For this review, use the dimensioned drawing (mm, ordinates from the lowest corner) and the shaded views. Give positions to 0.01 mm unless a question says otherwise; leave off trailing zeros. Write each loop counter-clockwise with the first axis right and the second up, starting at its lowest first coordinate (ties: lowest second). Pieces come first, ordered by that corner, then holes. Notation, with made-up numbers: (87.5, -7) -> (140.5, -7) arc R17 ccw to (140.5, 17) -> close; hole circle Ø5 at (81.5, 27.25). An arc over 180 degrees is marked (long way). Answer as CSV lines item,"result".
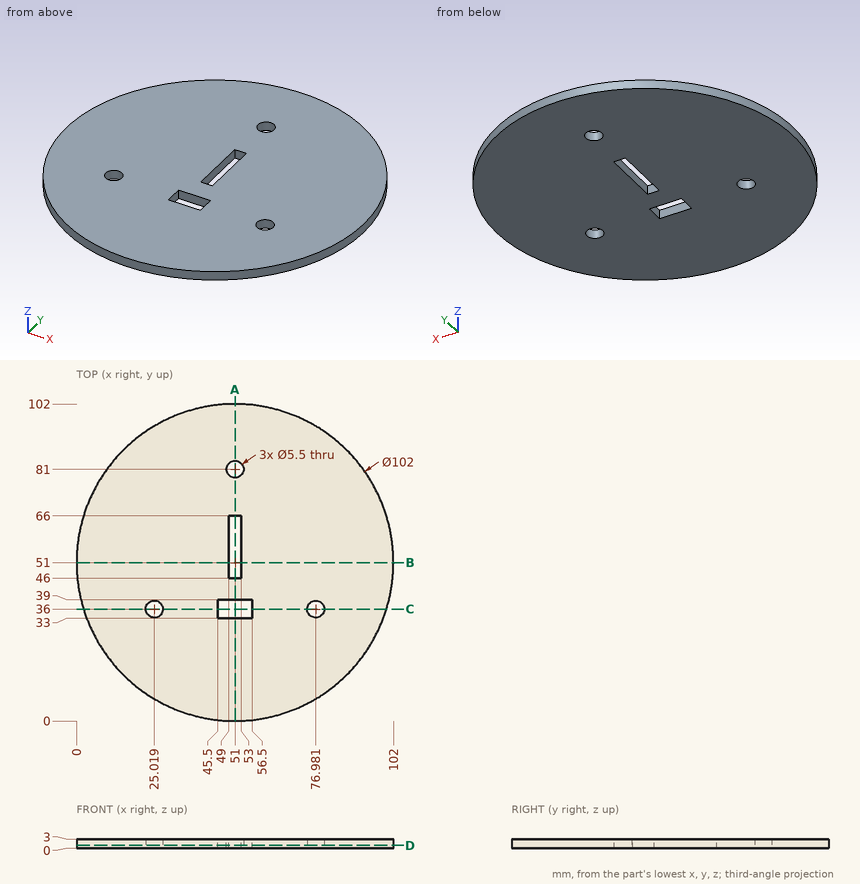
Q1. Clearance check with flat-ended pins moving along their axes: pin 1 (1.5 mm diameter, centred on x = 30, z = 0.5, fed in from +Y); pin 2 (0.9 mm diameter, centred on x = 51, z = 2, fed in from -Y); pin 3 (1 mm diameter, centred on x = 73, z = 1.5, fed in from -Y). State where each tip first meets the part, or that it passes through.
Answer block:
pin 1,"stops at y = 97.81"
pin 2,"stops at y = 0"
pin 3,"stops at y = 4.75"
Q2. Add section D-D (z = 0.95). Write out the cut boundary in (x, y), plus the area to 3 significant figures.
Answer block:
outline,"circle Ø102 at (51, 51); hole circle Ø5.5 at (25.02, 36); hole (45.5, 33) -> (56.5, 33) -> (56.5, 39) -> (45.5, 39) -> close; hole circle Ø5.5 at (51, 81); hole (49, 46) -> (53, 46) -> (53, 66) -> (49, 66) -> close; hole circle Ø5.5 at (76.98, 36)"
area,"7,950 mm2"
Q3. To check wall thickness, follow probe 1 along Y at (x, z) = (51, 2.4); probe 2 along X at (y, z) = (36.5, 1.45) (1 decimal); probe 3 along X at (y, z) = (48.5, 1.3). State the ranges of each line that lie inside material, in increasing order. Write a range as [from, to].
Answer block:
probe 1,"y = [0, 33], [39, 46], [66, 78.25], [83.75, 102]"
probe 2,"x = [2.1, 22.3], [27.7, 45.5], [56.5, 74.3], [79.7, 99.9]"
probe 3,"x = [0.06, 49], [53, 101.94]"
Q4. Add section A-A (x = 51). Write out the cut boundary in (y, z).
Answer block:
outline,"(0, 0) -> (33, 0) -> (33, 3) -> (0, 3) -> close; (39, 0) -> (46, 0) -> (46, 3) -> (39, 3) -> close; (66, 0) -> (78.25, 0) -> (78.25, 3) -> (66, 3) -> close; (83.75, 0) -> (102, 0) -> (102, 3) -> (83.75, 3) -> close"
Q5. Add section B-B (y = 51). Write out the cut boundary in (x, z), plus the area to 3 significant figures.
Answer block:
outline,"(0, 0) -> (49, 0) -> (49, 3) -> (0, 3) -> close; (53, 0) -> (102, 0) -> (102, 3) -> (53, 3) -> close"
area,"294 mm2"
Q6. Add section C-C (y = 36). Write out the cut boundary in (x, z).
Answer block:
outline,"(2.26, 0) -> (22.27, 0) -> (22.27, 3) -> (2.26, 3) -> close; (27.77, 0) -> (45.5, 0) -> (45.5, 3) -> (27.77, 3) -> close; (56.5, 0) -> (74.23, 0) -> (74.23, 3) -> (56.5, 3) -> close; (79.73, 0) -> (99.74, 0) -> (99.74, 3) -> (79.73, 3) -> close"
